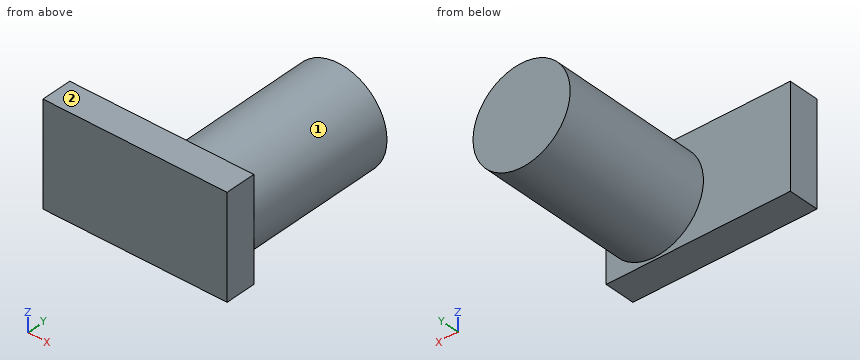
Autodesk Inventor part; units mm, degrees
ref_plane "YZ Plane" through (0, 0, 0) normal (1, 0, 0) x (0, 1, 0)
ref_plane "XZ Plane" through (0, 0, 0) normal (0, 1, 0) x (-1, 0, 0)
ref_plane "XY Plane" through (0, 0, 0) normal (0, 0, 1) x (1, 0, 0)
sketch "Sketch1" plane through (0, 0, 0) normal (0, 1, 0) x (-1, 0, 0)
  line L0 (9, 5) -> (-9, 5)
  line L1 (-9, 5) -> (-9, -5)
  line L2 (-9, -5) -> (9, -5)
  line L3 (9, -5) -> (9, 5)
  line L4 (9, 5) -> (-9, -5) construction
  line L5 (-9, 5) -> (9, -5) construction
  point P0 (0, 0)
  dimension "d0" = 18
  dimension "d1" = 10
extrude "Extrusion1" add sketch "Sketch1" along normal blind 3
sketch "Sketch2" plane through (0, 3, 0) normal (0, 1, 0) x (1, 0, 0)
  circle A0 centre (4.25, 0) radius 4.75
  line L0 (9, -5) -> (9, 5)
  point P0 (0, 0)
  dimension "d4" = 9.5
extrude "Extrusion2" add sketch "Sketch2" along normal blind 15
properties part number "Candado"
Work out the finished part from the listing and answer in its coordinate system (mm). Face numbers are marked on the shaded views. A direction names the side the tool comes from. Round coordinates to 2 decimals unless told otherwise and drop trailing zeros. Write each loop counter-clockwise with the first axis right and the second up, starting at its lowest first coordinate (ties: lowest second). Pieces come first, ordered by that corner, then holes.
1) A cutting plane is placed at C-C on y = 11. Determine the outline of the cut face in (x, z), and give its area (3 significant figures).
2) A cutting plane is placed at B-B on z = 1.75. Determine the outline of the cut face in (x, y).
3) Which of the six approach directions +Z, -Z, +X, -X, +Y, -Y give full straight-line access (tool end or side, diameter ignored) to the marked faces 1 and 2?
4) Flat-ended cylindrical pins translate along their axes: P1, Ø6, axis at x = 7, y = 9.5, coming from the -Z side; P2, Ø1.5, axis at y = 7.5, z = 4, coming from the -X side. Find the tip coordinate at first contact, or state that the pin passes through.
5) A cutting plane is placed at D-D on x = -5. Determine the outline of the cut face in (y, z), and give its area (3 significant figures).
6) Consider probe 1 along X at (y, z) = (14, 0); probe 2 along Y at (x, z) = (0.5, -4); probe 3 along Z at (x, y) = (4, 5). Determine where each line is inside the solid, lowest interval first.
7) A cutting plane is placed at A-A on x = 4.25. Determine the outline of the cut face in (y, z).
Entries:
1. outline: circle Ø9.5 at (4.25, 0)
1. area: 70.9 mm2
2. outline: (-9, 0) - (9, 0) - (9, 3) - (8.67, 3) - (8.67, 18) - (-0.17, 18) - (-0.17, 3) - (-9, 3) - close
3. face 1: +Y
3. face 2: +Z, +X, -X, +Y, -Y
4. P1: stops at z = -4.75
4. P2: stops at x = 0.79
5. outline: (0, -5) - (3, -5) - (3, 5) - (0, 5) - close
5. area: 30.0 mm2
6. probe 1: x = -0.5 to 9
6. probe 2: y = 0 to 3
6. probe 3: z = -4.74 to 4.74
7. outline: (0, -5) - (3, -5) - (3, -4.75) - (18, -4.75) - (18, 4.75) - (3, 4.75) - (3, 5) - (0, 5) - close
